Could you check a few things on this drawing? It's one solid part, dimensions in mm from its lowest x, y, z. A direction names the side the tool comes from. Round coordinates to 2 decimals unless told otherwise and drop trailing zeros. Write each loop counter-clockwise with the first axis right and the second up, starting at its lowest first coordinate (ties: lowest second). Pieces come first, ordered by that corner, then holes. Notation, with made-up numbers: (66.5, 9) - (77.5, 9) arc R16 ccw to (77.5, 15) - close; hole circle Ø1 at (9, 2). An arc over 180 degrees is marked (long way). One line per question, with ' | ' between items. Start each with the question number.
(1) For the marked faces 4, 5, 6 and 7, which set-ups out of +Z, -Z, +X, -X, +Y, -Y let a thin tool reach every point of the face, with its end or its side?
(2) Imagine slicing it at C-C (x = 18.5). Write out the boundary of the cut face in (y, z), plus the area to 3 significant figures.
(3) Imagine slicing it at A-A (z = 34). Write out the boundary of the cut face in (x, y), plus the area to 3 significant figures.
(4) Imagine slicing it at B-B (z = 16). Write out the boundary of the cut face in (x, y), plus the area to 3 significant figures.
(5) Will these pins go through, and if not, where does the flat tip stop? pin 1 (5 mm diameter, centred on y = 20, z = 16, fed in from +X); pin 2 (1 mm diameter, centred on x = 8, y = 10, fed in from +Z); pin 3 (2 mm diameter, centred on x = 3, y = 21.5, fed in from -Z); pin 4 (4.5 mm diameter, centred on x = 9, z = 14.5, fed in from +Y).
(6) Imagine slicing it at D-D (y = 4). Give the number of separate pieces and of enclosed holes in the cut face, plus the area to 3 significant figures.
(7) Thinking about a two-plate mould opening in Z: for the marked faces 1, 2 and 3, which applies, pulls with the +Z half, pulls with the -Z half, needs draft (parallel to the pull), parting line crosses it, or undercut?
(8) If I drill on L1, parallel to Z at x = 17.5, y = 4; L2, parallel to Z at x = 3, y = 20; L3, parallel to Y at x = 15.25, z = 4, over which ranges is the centre line in solid material (lowest first)?
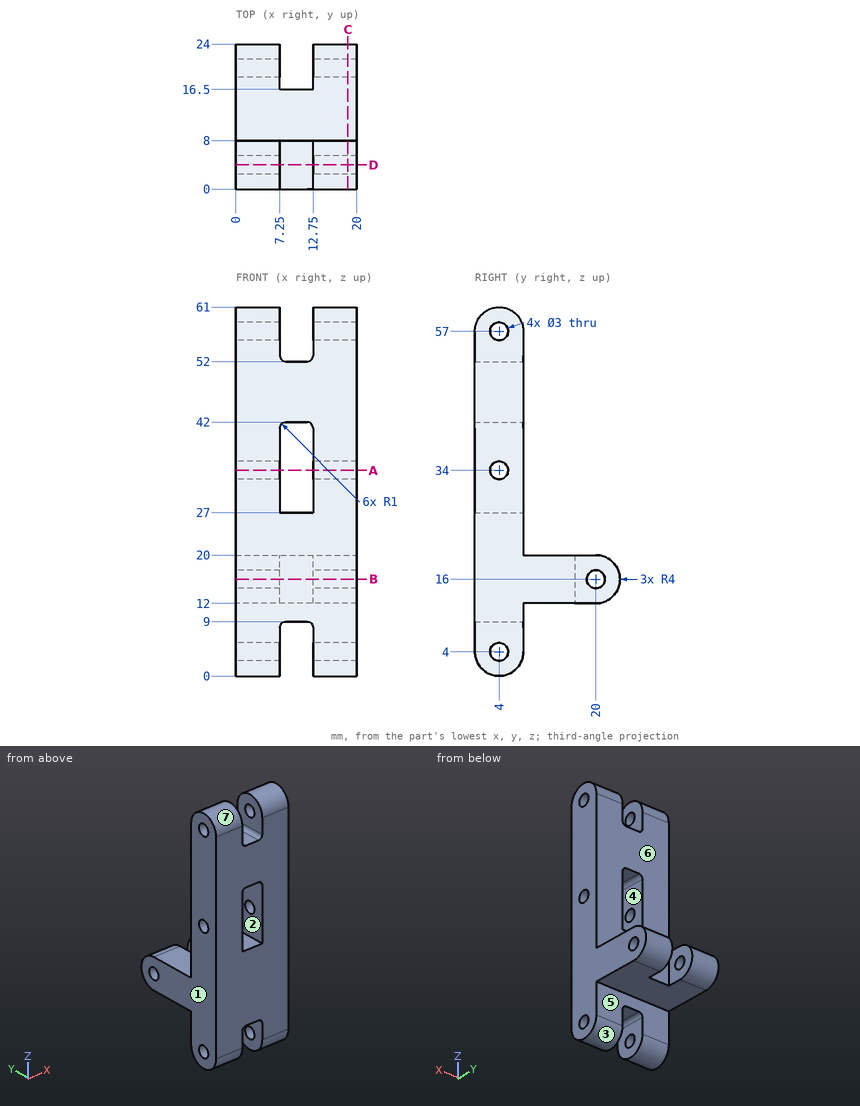
Check sheet entries:
1) face 4: +Y, -Y | face 5: -Z, +X, -X, +Y | face 6: +Z, +X, -X, +Y | face 7: +Z, +X, -X
2) outline: (0, 4) arc R4 ccw to (8, 4) - (8, 12) - (20, 12) arc R4 ccw to (20, 20) - (8, 20) - (8, 57) arc R4 ccw to (0, 57) - close; hole circle Ø3 at (4, 4); hole circle Ø3 at (4, 34); hole circle Ø3 at (4, 57); hole circle Ø3 at (20, 16) | area: 567 mm^2
3) outline: (0, 0) - (7.25, 0) - (7.25, 2.5) - (0, 2.5) - close; (0, 5.5) - (7.25, 5.5) - (7.25, 8) - (0, 8) - close; (12.75, 0) - (20, 0) - (20, 2.5) - (12.75, 2.5) - close; (12.75, 5.5) - (20, 5.5) - (20, 8) - (12.75, 8) - close | area: 72.5 mm^2
4) outline: (0, 0) - (20, 0) - (20, 18.5) - (12.75, 18.5) - (12.75, 16.5) - (7.25, 16.5) - (7.25, 18.5) - (0, 18.5) - close; (0, 21.5) - (7.25, 21.5) - (7.25, 24) - (0, 24) - close; (12.75, 21.5) - (20, 21.5) - (20, 24) - (12.75, 24) - close | area: 395 mm^2
5) pin 1: x = 20 | pin 2: z = 20 | pin 3: z = 12.03 | pin 4: y = 24
6) separate pieces: 6 | enclosed holes: 0 | area: 909 mm^2
7) face 1: needs draft | face 2: undercut | face 3: pulls with the -Z half
8) L1: 0 to 2.5, 5.5 to 32.5, 35.5 to 55.5, 58.5 to 61 | L2: 12 to 14.5, 17.5 to 20 | L3: 0 to 2.5, 5.5 to 8
